The listing builds one solid part. Answer for the finished solid, in the listing's coordinates (mm). A direction names the side the tool comes from. Round coordinates to 2 decimals unless told otherwise and drop trailing zeros. Write each loop counter-clockwise with the first axis right and the second up, starting at its lowest first coordinate (ties: lowest second). Pieces come first, ordered by that corner, then holes.
(1) The mould has two halves that part along X. Classify faces 6 (the face through (11, 5, 6)), 7 (the face through (-8, 0, 6)), 8 (the face through (3, 0, 12)): +X half, -X half, draft (parallel to the pull), parting line (faces both ways), or undercut.
(2) A cutting plane is placed at A-A, the plane z = 6. Give the vertices of the cut face in (x, y), and give its area (3 significant figures).
(3) For faces 1 (the face through (6, 0, 10)), 2 (the face through (11, 6, 7)), 3 (the face through (6, 8, 6)), 4 (the face through (6.16, -7.43, 11.4)), 5 (the face through (5.5, 0, 6)), determine the directions among +Z, -Z, +X, -X, +Y, -Y from which every point of the face is accessible in a straight line to the end or side of a thin tool.
(4) A cutting plane is placed at B-B, the plane y = 0. Give the vertices of the cut face in (x, z), and give its area (3 significant figures).
(5) Find the intervals of material crossed by probe 1 along Z at (x, y) = (12.5, -5.5); probe 2 along Y at (x, z) = (8, 3.75); probe 3 along X at (y, z) = (5, 6) (3 decimals), in increasing order.
(6) A cutting plane is placed at C-C, the plane x = 7.75. Give the vertices of the cut face in (y, z), and give its area (3 significant figures).
(7) Each of these flat-tipped pins is pushed along its axis until it touches: pin 1 Ø3 at (y, z) = (-5, 9.5) entering from -X; pin 2 Ø1 at (y, z) = (-1.5, 1) entering from +X; pin 3 Ø5 at (y, z) = (-2.5, 3) entering from +X. Where does it stop, or does it pass through?
Autodesk Inventor part; units mm, degrees
ref_plane "YZ Plane" through (0, 0, 0) normal (1, 0, 0) x (0, 1, 0)
ref_plane "XZ Plane" through (0, 0, 0) normal (0, 1, 0) x (-1, 0, 0)
ref_plane "XY Plane" through (0, 0, 0) normal (0, 0, 1) x (1, 0, 0)
sketch "Sketch2" plane through (0, 0, 0) normal (0, 0, 1) x (1, 0, 0)
  circle A0 centre (0, 0) radius 1.75
  circle A1 centre (0, 0) radius 8 construction
  arc A2 (0, 8) -> (0, -8) centre (0, 0) ccw
  line L0 (0, 8) -> (6, 8)
  line L1 (6, 8) -> (6, -8)
  line L2 (6, -8) -> (0, -8)
  dimension "d0" = 3.5
  dimension "d1" = 16
  dimension "d2" = 6
extrude "Extrusion1" add sketch "Sketch2" along normal blind 12
sketch "Sketch3" plane through (0, -8, 0) normal (0, -1, 0) x (1, 0, 0)
  circle A0 centre (12.5, 6) radius 6 construction
  line L0 (6, 0) -> (6, 12)
  line L1 (0, 0) -> (0, 12)
  circle A1 centre (12.5, 6) radius 1.5
  arc A2 (12.5, 0) -> (12.5, 12) centre (12.5, 6) ccw
  line L2 (6, 12) -> (12.5, 12)
  line L3 (6, 0) -> (12.5, 0)
  point P0 (6, 6)
  dimension "d5" = 12
  dimension "d6" = 12.5
  dimension "d7" = 3
extrude "Extrusion2" add sketch "Sketch3" against normal blind 5
sketch "Sketch4" plane through (0, 8, 0) normal (0, 1, 0) x (1, 0, 0)
  circle A0 centre (12.5, -6) radius 1.5
  line L0 (6, -12) -> (6, 0)
  line L1 (6, -12) -> (12.5, -12)
  arc A1 (12.5, -12) -> (12.5, 0) centre (12.5, -6) ccw
  line L2 (12.5, 0) -> (6, 0)
  point P0 (0, 0)
extrude "Extrusion3" add sketch "Sketch4" against normal blind 5
sketch "Sketch6" plane through (0, 8, 12) normal (0, 1, 0) x (1, 0, 0)
  circle A0 centre (12.5, 6) radius 1.5
  circle A1 centre (12.5, 6) radius 3
  point P0 (0, 12)
  dimension "d13" = 6
extrude "Extrusion4" cut sketch "Sketch6" against normal blind 2
sketch "Sketch7" plane through (0, -3, 0) normal (0, 1, 0) x (1, 0, 0)
  arc A0 (12.5, -12) -> (12.5, 0) centre (12.5, -6) ccw
  circle A1 centre (12.5, -6) radius 7
  point P0 (0, 0)
  dimension "d16" = 14
extrude "Extrusion5" cut sketch "Sketch7" along normal blind 6
fillet "Fillet1" radius 2 8 edges at (18.5, 8, 6) (6.25, 8, 0) (-8, 0, 0) (6.25, -8, 0) (18.5, -8, 6) (6.25, -8, 12) (-8, 0, 12) (6.25, 8, 12)
properties part number "Arm1" material "ABS Plastic"
Solutions:
1. face 6: undercut
1. face 7: -X half
1. face 8: draft
2. outline: (0, -8) - (11, -8) - (11, -3) - (5.5, -3) - (5.5, 3) - (11, 3) - (11, 6) - (9.5, 6) - (9.5, 8) - (0, 8) arc R8 ccw to start; (14, -8) - (16.5, -8) arc R2 ccw to (18.5, -6) - (18.5, -3) - (14, -3) - close; (14, 3) - (18.5, 3) - (18.5, 6) arc R2 ccw to (16.5, 8) - (15.5, 8) - (15.5, 6) - (14, 6) - close; hole circle Ø3.5 at (0, 0)
2. area: 271 mm2
3. face 1: +Z, -Z, +X
3. face 2: +Y
3. face 3: +Z, -Z, +X, -X, +Y
3. face 4: +Z, +X, -X, -Y
3. face 5: +X
4. outline: (-8, 2) arc R2 ccw to (-6, 0) - (-1.75, 0) - (-1.75, 12) - (-6, 12) arc R2 ccw to (-8, 10) - close; (1.75, 0) - (6, 0) - (6, 3.4) arc R7 cw to (6, 8.6) - (6, 12) - (1.75, 12) - close
4. area: 123 mm2
5. probe 1: z = 0 to 4.5, 7.5 to 12
5. probe 2: y = -8 to -3, 3 to 8
5. probe 3: x = -6.245 to 11, 14 to 18.5
6. outline: (-8, 2) arc R2 ccw to (-6, 0) - (-3, 0) - (-3, 12) - (-6, 12) arc R2 ccw to (-8, 10) - close; (3, 0) - (6, 0) arc R2 ccw to (8, 2) - (8, 10) arc R2 ccw to (6, 12) - (3, 12) - close
6. area: 117 mm2
7. pin 1: stops at x = -7.19
7. pin 2: stops at x = 6
7. pin 3: stops at x = 18.47
